Geometry check sheet. Reference: the model listing, model coordinates, mm. A direction names the side the tool comes from. Round coordinates to 2 decimals unless told otherwise and drop trailing zeros. Order: outer loops, then holes, each group sorted by start corner. A loop starts at its lowest first (then second) coordinate and runs counter-clockwise, first axis right, second up.
```python
from build123d import *

# Parameters (mm, degrees)
ESTRUSIONE_ESTRUSIONE1_DEPTH = 5
SCHIZZO3_R                   = 1.5
SCHIZZO3_RX                  = 23.25
SCHIZZO3_RY                  = 10
TAGLIO_ESTRUSIONE1_DEPTH     = 6
TAGLIO_ESTRUSIONE2_DEPTH     = 6.0000001
SCHIZZO6_W                   = 5
SCHIZZO6_H                   = 18
ESTRUSIONE_ESTRUSIONE2_DEPTH = 3


with BuildPart() as part:
    # Schizzo1 → Estrusione-Estrusione1 (new body)
    with BuildSketch(Plane(origin=(0, 0, 0), x_dir=(0, 0, -1), z_dir=(1, 0, 0))):
        Polygon((-113.645, -10), (113.645, -10), (113.645, 10), (-40.095, 10), (-40.095, 13), (-58.095, 13), (-58.095, 10), (-113.645, 10), align=None)
    extrude(amount=ESTRUSIONE_ESTRUSIONE1_DEPTH)

    # Schizzo3 → Taglio-Estrusione1 (cut, through all)
    with BuildSketch(Plane(origin=(0, 0, 0), x_dir=(0, 0, -1), z_dir=(1, 0, 0))):
        with Locations((-58.095, 5)):
            Circle(SCHIZZO3_R)
        with Locations((-72.345, 5)):
            Circle(SCHIZZO3_R)
        with Locations((-40.095, 5)):
            Circle(SCHIZZO3_R)
        with Locations((-25.845, 5)):
            Circle(SCHIZZO3_R)
        with Locations((14.155, 5)):
            Circle(SCHIZZO3_R)
        with Locations((54.155, 5)):
            Circle(SCHIZZO3_R)
        with Locations((94.155, 5)):
            Circle(SCHIZZO3_R)
        with Locations((-102.345, 5)):
            Circle(SCHIZZO3_R)
        with Locations(Location((-49.095, -10), (0, 0, 0))):
            Ellipse(SCHIZZO3_RX, SCHIZZO3_RY)
    extrude(amount=TAGLIO_ESTRUSIONE1_DEPTH, mode=Mode.SUBTRACT)

    # Schizzo5 → Taglio-Estrusione2 (cut, through all)
    with BuildSketch(Plane(origin=(0, 0, 0), x_dir=(0, 0, -1), z_dir=(1, 0, 0))):
        Polygon((-88.595, 0), (-88.595, 3.8), (-90.095, 3.8), (-90.095, 6.2), (-88.595, 6.2), (-88.595, 10), (-86.095, 10), (-86.095, 6.2), (-84.595, 6.2), (-84.595, 3.8), (-86.095, 3.8), (-86.095, 0), align=None)
        Polygon((-7.095, 0), (-7.095, 3.8), (-8.595, 3.8), (-8.595, 6.2), (-7.095, 6.2), (-7.095, 10), (-4.595, 10), (-4.595, 6.2), (-3.095, 6.2), (-3.095, 3.8), (-4.595, 3.8), (-4.595, 0), align=None)
        Polygon((72.905, 0), (72.905, 3.8), (71.405, 3.8), (71.405, 6.2), (72.905, 6.2), (72.905, 10), (75.405, 10), (75.405, 6.2), (76.905, 6.2), (76.905, 3.8), (75.405, 3.8), (75.405, 0), align=None)
    extrude(amount=TAGLIO_ESTRUSIONE2_DEPTH, mode=Mode.SUBTRACT)

    # Schizzo6 → Estrusione-Estrusione2 (add)
    with BuildSketch(Plane(origin=(0, 10, 0), x_dir=(1, 0, 0), z_dir=(0, 1, 0))):
        with Locations((2.5, 47.225)):
            Rectangle(SCHIZZO6_W, SCHIZZO6_H)
    extrude(amount=ESTRUSIONE_ESTRUSIONE2_DEPTH)


solid = part.part
```
(1) Sectioned sample at A-A, the plane x = 3.3. Give the number of separate pieces and of enclosed holes in the cut face, and give its area (3 significant figures).
Returned:
separate pieces: 1
enclosed holes: 8
area: 4,140 mm2
(2) Set-up check for faces 1 (the flat face through (2, 10, -95)), 2 (the flat face through (2, 2, 7.095)), 3 (the flat face through (2, -10, -43)), 4 (the flat face through (0, 2, 2)), 5 (the flat face through (2, 10, 72)): record each of +Z, -Z, +X, -X, +Y, -Y from which the full face is reachable in a straight line by a thin tool's end or side.
Returned:
face 1: -Z, +X, -X, +Y
face 2: +X, -X, +Y
face 3: +Z, -Z, +X, -X, -Y
face 4: +Z, -Z, -X, +Y, -Y
face 5: +Z, +X, -X, +Y
(3) Sectioned sample at B-B, the plane z = 11. Record the cut outline in (x, y), and give its area (3 significant figures).
Returned:
outline: (0, -10) - (5, -10) - (5, 10) - (0, 10) - close
area: 100 mm2
(4) Draft check along Z on faces 6 (the flat face through (2, 2, 86.095)), 7 (the flat face through (2, 13, -47)), 8 (the flat face through (2, 0, -113.645)). Enter one of: released by +Z, released by -Z, zero draft, split by the parting line, or undercut.
Returned:
face 6: undercut
face 7: zero draft
face 8: released by -Z
(5) Depth check by flat-ended pin: P1, Ø1.5, axis at x = 1.5, y = 11, coming from the -Z side (3 decimals); P2, Ø10, axis at y = 1.5, z = 71.5, coming from the -X side; P3, Ø1.5, axis at x = 3, y = 12, coming from the +Z side (3 decimals); P4, Ø3, axis at x = 3, z = -13.5, coming from the +Y side. Enter the tip coordinate at first touch or a pass-through.
Returned:
P1: stops at z = -56.225
P2: stops at x = 0
P3: stops at z = 58.095
P4: stops at y = 10
(6) Material ranges on line 1 (Z direction, x = 2.4, y = 9) (3 decimals); line 2 (Y direction, x = 4.1, z = -94.5); line 3 (Z direction, x = 4.3, y = -6.5) (3 decimals), recorded low to high.
Returned:
line 1: z = -113.645 to -75.405, -72.905 to 4.595, 7.095 to 86.095, 88.595 to 113.645
line 2: y = -10 to 3.54, 6.46 to 10
line 3: z = -113.645 to 27.316, 70.874 to 113.645
